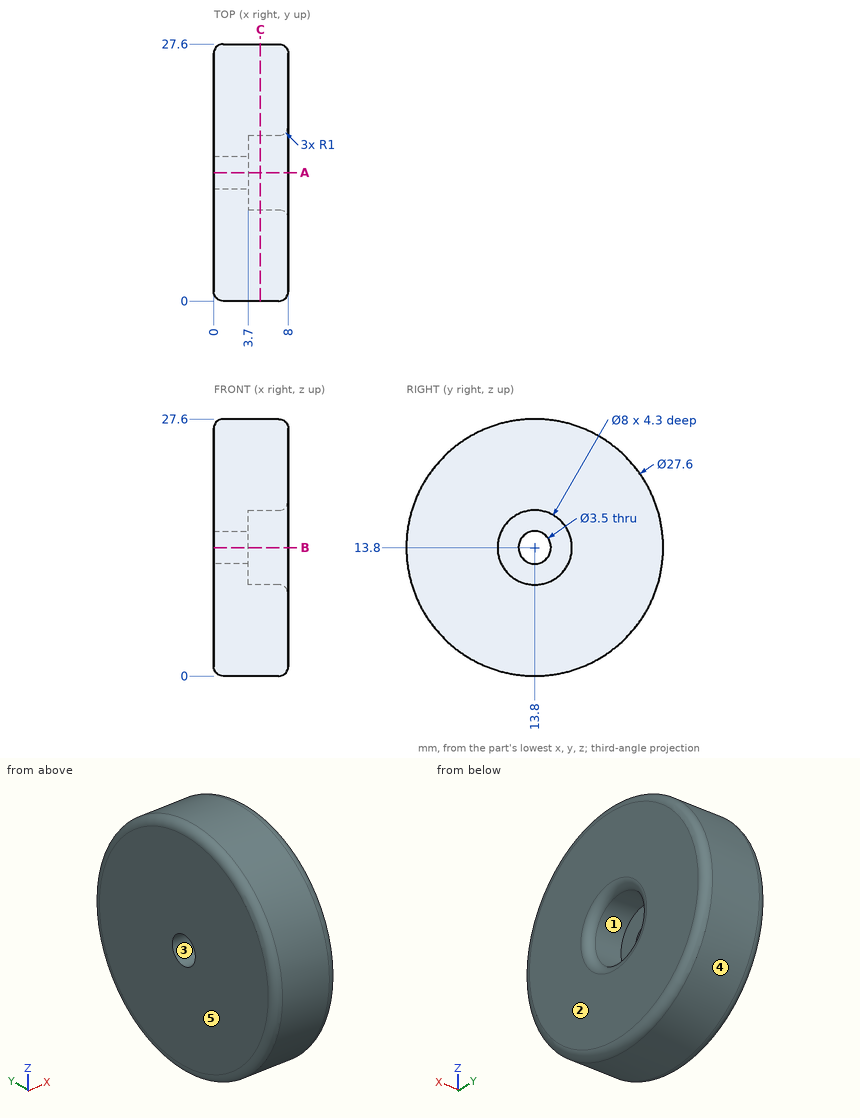
Study the drawing (mm; zero at the part's minimum x, y, z) and answer. A direction names the side the tool comes from. Round coordinates to 2 decimals unless told otherwise and drop trailing zeros. Loops run counter-clockwise (first coordinate to the right, second up) from the corner with the lowest first, then second, coordinate; pieces in that order, holes last. Notation, with made-up numbers: (82.5, 64.5) -> (90.5, 64.5) arc R36 cw to (90.5, 102.5) -> close; hole circle Ø7 at (7, -38.5). An arc over 180 degrees is marked (long way). One line per item, written item: value.
1) Flat-ended cylindrical pins translate along their axes: P1, Ø4, axis at y = 13.8, z = 13.8, coming from the +X side; P2, Ø3, axis at x = 3.5, z = 20, coming from the -Y side (3 decimals). Find the tip coordinate at first contact, or state that the pin passes through.
Answer list:
P1: stops at x = 3.7
P2: stops at y = 0.825
2) A cutting plane is placed at A-A (y = 13.8). Determine the outline of the cut face in (x, z).
Answer list:
outline: (0, 1) arc R1 ccw to (1, 0) -> (7, 0) arc R1 ccw to (8, 1) -> (8, 8.8) arc R1 ccw to (7, 9.8) -> (3.7, 9.8) -> (3.7, 12.05) -> (0, 12.05) -> close; (0, 15.55) -> (3.7, 15.55) -> (3.7, 17.8) -> (7, 17.8) arc R1 ccw to (8, 18.8) -> (8, 26.6) arc R1 ccw to (7, 27.6) -> (1, 27.6) arc R1 ccw to (0, 26.6) -> close
3) The mould has two halves that part along Z. Classify the marked faces 3, 4 and 5: pulls with the +Z half, pulls with the -Z half, needs draft (parallel to the pull), parting line crosses it, or undercut.
Answer list:
face 3: undercut
face 4: parting line crosses it
face 5: needs draft
4) A cutting plane is placed at C-C (x = 5). Determine the outline of the cut face in (y, z).
Answer list:
outline: circle Ø27.6 at (13.8, 13.8); hole circle Ø8 at (13.8, 13.8)
5) Consider L1, parallel to Z at x = 4, y = 14.25; L2, parallel to Z at x = 5.25, y = 12; L3, parallel to Z at x = 5, y = 2.75. Determine where each line is inside the solid, lowest interval first. Write a range as [from, to].
Answer list:
L1: z = [0.01, 9.83], [17.77, 27.59]
L2: z = [0.12, 10.23], [17.37, 27.48]
L3: z = [5.53, 22.07]
6) For the marked faces 1 and 2, determine the directions among +Z, -Z, +X, -X, +Y, -Y from which every point of the face is accessible in a straight line to the end or side of a thin tool.
Answer list:
face 1: +X
face 2: +Z, -Z, +X, +Y, -Y
